Model file for the job. Use its own axes, mm. Face numbers are marked on the shaded views. Round coordinates to 2 decimals unless told otherwise and drop trailing zeros. Loops run counter-clockwise (first coordinate to the right, second up) from the corner with the lowest first, then second, coordinate; pieces in that order, holes last.
from build123d import *

# Parameters (mm, degrees)
SKETCH1_R           = 1.9
BOSS_EXTRUDE1_DEPTH = 1.6
CHAMFER1_SIZE       = 0.2


with BuildPart() as part:
    # Sketch1 → Boss-Extrude1 (new, symmetric)
    with BuildSketch(Plane(origin=(0, 0, 0), x_dir=(1, 0, 0), z_dir=(0, 1, 0))):
        Polygon((4.041451884, 0), (2.020725942, 3.5), (-2.020725942, 3.5), (-4.041451884, 0), (-2.020725942, -3.5), (2.020725942, -3.5), align=None)
        with Locations(Location((0, 0, 0), (0, 0, 270))):
            Circle(SKETCH1_R, mode=Mode.SUBTRACT)
    extrude(amount=BOSS_EXTRUDE1_DEPTH, both=True)

    # Sketch2 → Cut-Revolve1 (revolve, cut)
    with BuildSketch(Plane.XY):
        with BuildLine():
            Line((-4.3, -0.8), (-4.3, -1.6))
            Line((-4.3, -1.6), (-3.5, -1.6))
            ThreePointArc((-3.5, -1.6), (-4.065685425, -1.365685425), (-4.3, -0.8))
        make_face()
    cut_revolve1 = revolve(axis=Axis((0, 0, 0), (0, 1, 0)), mode=Mode.SUBTRACT)

    # Mirror2: Cut-Revolve1 across plane
    add(cut_revolve1.mirror(Plane.ZX), mode=Mode.SUBTRACT)

    # Chamfer1
    chamfer1_edges = [part.edges().sort_by_distance(p)[0] for p in [
        (0, -1.6, -1.9),
        (0, 1.6, -1.9),
    ]]
    chamfer(chamfer1_edges, length=CHAMFER1_SIZE)


solid = part.part
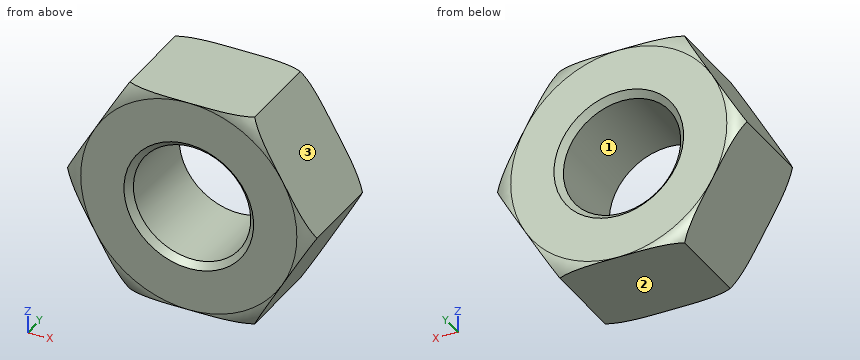
Q1. Slice it at A-A on y = -0.75. Give the cut face in (x, z).
Q2. Probe line 1 (X direction, y = 0.6, z = 1.5); line 2 (X direction, y = -0.8, z = 1); line 3 (Z direction, x = 0.75, y = -1.25). List the from-to ranges inside material, lowest first.
Q3. Pull direction Z, two halves, no side cores. Call the marked faces 1, 2 and 3: pulls with the +Z half, pulls with the -Z half, needs draft (parallel to the pull), parting line crosses it, or undercut.
Reply:
1. outline: (-4.04, 0) - (-2.02, -3.5) - (2.02, -3.5) - (4.04, 0) - (2.02, 3.5) - (-2.02, 3.5) - close; hole circle Ø3.8 at (0, 0)
2. line 1: x = -3.18 to -1.17, 1.17 to 3.18
2. line 2: x = -3.46 to -1.62, 1.62 to 3.46
2. line 3: z = -3.5 to -1.75, 1.75 to 3.5
3. face 1: undercut
3. face 2: pulls with the -Z half
3. face 3: pulls with the +Z half
